from build123d import *

# Parameters (mm, degrees)
SKETCH2_R           = 1.6
BOSS_EXTRUDE1_DEPTH = 1.5


with BuildPart() as part:
    # Sketch2 → Boss-Extrude1 (new body)
    with BuildSketch(Plane(origin=(0, 0, 0), x_dir=(1, 0, 0), z_dir=(0, 1, 0))):
        with BuildLine():
            ThreePointArc((-18.257935671, 38.931321388), (-30.460746389, 30.350336562), (-38.99736345, 18.116446781))
            ThreePointArc((-38.99736345, 18.116446781), (-31.450297137, -0.057101793), (-38.931321388, -18.257935671))
            ThreePointArc((-38.931321388, -18.257935671), (-30.350336562, -30.460746389), (-18.116446781, -38.99736345))
            ThreePointArc((-18.116446781, -38.99736345), (0.057101793, -31.450297137), (18.257935671, -38.931321388))
            ThreePointArc((18.257935671, -38.931321388), (30.460746389, -30.350336562), (38.99736345, -18.116446781))
            ThreePointArc((38.99736345, -18.116446781), (31.450297137, 0.057101793), (38.931321388, 18.257935671))
            ThreePointArc((38.931321388, 18.257935671), (30.350336562, 30.460746389), (18.116446781, 38.99736345))
            ThreePointArc((18.116446781, 38.99736345), (-0.057101793, 31.450297137), (-18.257935671, 38.931321388))
        make_face()
        with Locations((19.75, 34.208003449)):
            Circle(SKETCH2_R, mode=Mode.SUBTRACT)
        with Locations((34.208003449, 19.75)):
            Circle(SKETCH2_R, mode=Mode.SUBTRACT)
        with Locations((19.75, -34.208003449)):
            Circle(SKETCH2_R, mode=Mode.SUBTRACT)
        with Locations((34.208003449, -19.75)):
            Circle(SKETCH2_R, mode=Mode.SUBTRACT)
        with Locations((-34.208003449, -19.75)):
            Circle(SKETCH2_R, mode=Mode.SUBTRACT)
        with Locations((-19.75, -34.208003449)):
            Circle(SKETCH2_R, mode=Mode.SUBTRACT)
        with Locations((-19.75, 34.208003449)):
            Circle(SKETCH2_R, mode=Mode.SUBTRACT)
        with Locations((-34.208003449, 19.75)):
            Circle(SKETCH2_R, mode=Mode.SUBTRACT)
        with Locations((-18.257935671, 18.116446781)):
            Circle(SKETCH2_R, mode=Mode.SUBTRACT)
        with Locations((18.257935671, 18.116446781)):
            Circle(SKETCH2_R, mode=Mode.SUBTRACT)
        with Locations((-18.257935671, -18.257935671)):
            Circle(SKETCH2_R, mode=Mode.SUBTRACT)
        with Locations((18.257935671, -18.257935671)):
            Circle(SKETCH2_R, mode=Mode.SUBTRACT)
    extrude(amount=BOSS_EXTRUDE1_DEPTH)


solid = part.part
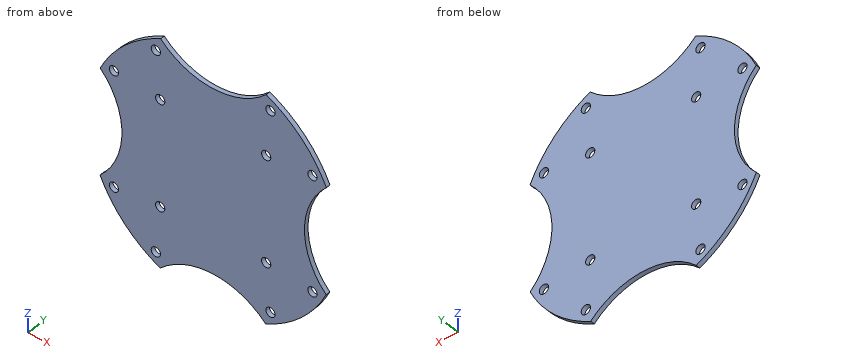
Model file for the job. Use its own axes, mm. Give positions to 0.01 mm unless a question says otherwise; leave off trailing zeros. Order: outer loops, then holes, each group sorted by start corner. A loop starts at its lowest first (then second) coordinate and runs counter-clockwise, first axis right, second up. Notation, with made-up numbers: (-34, 53.5) - (-1, 53.5) arc R5 cw to (-1, 60.5) - close; hole circle Ø11 at (-15, -39). An arc over 180 degrees is marked (long way). Write item = value, one per line. Start each with the question number.
1. Cut at C-C, the plane x = -15. List the corners of the cut face in (y, z).
2. Cut at A-A, the plane y = 0.3. State how many separate pieces and enclosed holes the cut face has, and give its area (3 significant figures).
3. Drop flat-ended pins along their axis: P1, Ø3, axis at x = 18.26, z = -18.12, coming from the +Y side; P2, Ø5, axis at x = -18.26, z = 18.26, coming from the -Y side. Give the stop position or say it passes through.
4. Cut at B-B, the plane z = -4.5. List the corners of the cut face in (x, y), and give its area (3 significant figures).
5. Probe line 1 along Z through (x, y) = (17.5, 1.35); line 2 along X through (y, z) = (0.2, 18.5); line 3 along X through (y, z) = (0.95, 0). List the from-to ranges inside material, lowest first.
Taken from the geometry:
q1.outline = (0, -36.19) - (1.5, -36.19) - (1.5, 36.34) - (0, 36.34) - close
q2.separate_pieces = 1
q2.enclosed_holes = 12
q2.area = 4,560 mm²
q3.P1 = through
q3.P2 = 0
q4.outline = (-31.86, 0) - (31.83, 0) - (31.83, 1.5) - (-31.86, 1.5) - close
q4.area = 95.5 mm²
q5.line_1 = -38.4 to -19.53, -16.71 to 16.85, 19.67 to 38.21
q5.line_2 = -38.82 to -35.21, -33.21 to -19.84, -16.68 to 16.68, 19.84 to 33.21, 35.21 to 38.82
q5.line_3 = -31.45 to 31.45
